```python
from build123d import *

# Parameters (mm, degrees)
F0_W     = 300
F0_H     = 300
F1_DEPTH = 200
F2_W     = 297
F2_H     = 297
F3_DEPTH = 198.5
F5_DEPTH = 300
F6_W     = 280
F6_H     = 280
F7_DEPTH = 25


with BuildPart() as f1:
    # F0 (on Front) → F1 (new body)
    with BuildSketch(Plane.XZ):
        Rectangle(F0_W, F0_H)
    extrude(amount=F1_DEPTH)

    # F2 (on face) → F3 (cut)
    with BuildSketch(Plane.XZ.offset(200)):
        Rectangle(F2_W, F2_H)
    extrude(amount=-F3_DEPTH, mode=Mode.SUBTRACT)

    # F4 (on face) → F5 (join)
    with BuildSketch(Plane.YZ.offset(150)):
        Polygon((-174, 150), (-174, 0), (-174, -150), (-172.5, -150), (-172.5, 150), align=None)
    extrude(amount=-F5_DEPTH)

    # F6 (on face) → F7 (cut)
    with BuildSketch(Plane.XZ.offset(174)):
        Rectangle(F6_W, F6_H)
    extrude(amount=-F7_DEPTH, mode=Mode.SUBTRACT)


solid = f1.part
```
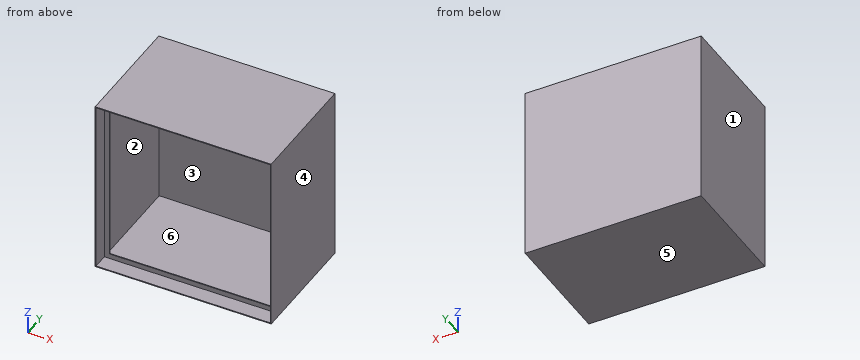
Check sheet for the modelled part. Datum: model origin and axes. Units: mm. Face numbers are marked on the shaded views. A direction names the side the tool comes from. Round coordinates to 2 decimals unless told otherwise and drop trailing zeros. Order: outer loops, then holes, each group sorted by start corner. A loop starts at its lowest first (then second) coordinate and runs counter-clockwise, first axis right, second up. Notation, with made-up numbers: (63.5, -14.5) -> (118.5, -14.5) arc R20 ccw to (118.5, -7.5) -> close; hole circle Ø8 at (-21.5, 28.25). An arc over 180 degrees is marked (long way). Use CSV: the item, a comma, the result in double quotes.
(1) Cross-section at A-A (z = 38). Record the boundary of the cut face in (x, y).
Worked out:
outline,"(-150, -200) -> (-148.5, -200) -> (-148.5, -174) -> (-140, -174) -> (-140, -172.5) -> (-148.5, -172.5) -> (-148.5, -1.5) -> (148.5, -1.5) -> (148.5, -172.5) -> (140, -172.5) -> (140, -174) -> (148.5, -174) -> (148.5, -200) -> (150, -200) -> (150, 0) -> (-150, 0) -> close"
(2) Cross-section at B-B (y = -167.5). Record the boundary of the cut face in (x, z), and give its area (3 significant figures).
Worked out:
outline,"(-150, -150) -> (150, -150) -> (150, 150) -> (-150, 150) -> close; hole (-148.5, -148.5) -> (148.5, -148.5) -> (148.5, 148.5) -> (-148.5, 148.5) -> close"
area,"1,790 mm²"
(3) Draft check along X on the marked faces 1, 2, 3 and 4. Enter one of: pulls with the +X half, pulls with the -X half, needs draft (parallel to the pull), parting line crosses it, or undercut.
Worked out:
face 1,"pulls with the -X half"
face 2,"undercut"
face 3,"undercut"
face 4,"pulls with the +X half"
(4) Cross-section at C-C (x = 33). Record the boundary of the cut face in (y, z), and give its area (3 significant figures).
Worked out:
outline,"(-200, -150) -> (0, -150) -> (0, 150) -> (-200, 150) -> (-200, 148.5) -> (-174, 148.5) -> (-174, 140) -> (-172.5, 140) -> (-172.5, 148.5) -> (-1.5, 148.5) -> (-1.5, -148.5) -> (-172.5, -148.5) -> (-172.5, -140) -> (-174, -140) -> (-174, -148.5) -> (-200, -148.5) -> close"
area,"1,070 mm²"
(5) Depth check by flat-ended pin: pin 1 (12 mm diameter, centred on x = 88.5, z = 90, fed in from -Y). Enter the tip coordinate at first touch or a pass-through.
Worked out:
pin 1,"y = -1.5"
(6) Material ranges on line 1 along Z through (x, y) = (-103, -177); line 2 along Y through (x, z) = (-45, -45), recorded low to high. Write a range as from..to.
Worked out:
line 1,"-150..-148.5, 148.5..150"
line 2,"-1.5..0"
(7) Tool access check on the marked faces 5 and 6. Record the directions out of +Z, -Z, +X, -X, +Y, -Y that give a thin tool (end or side, any length) a straight path to the whole face; none if there is none.
Worked out:
face 5,"-Z, +X, -X, +Y, -Y"
face 6,"none"
